```python
from build123d import *

# Parameters (mm, degrees)
SKETCH1_W                 = 254
SKETCH1_H                 = 114.3
BOSS_EXTRUDE1_DEPTH       = 5.08
CHAMFER1_SIZE             = 5.08
BOSS_EXTRUDE3_START       = -127
BOSS_EXTRUDE3_DEPTH       = 38.1
BOSS_EXTRUDE4_DEPTH       = 2.54
SKETCH6_R                 = 3
BOSS_EXTRUDE5_DEPTH       = 6
SKETCH12_R                = 3
SKETCH12_R_2              = 3.5
BOSS_EXTRUDE7_DEPTH       = 6
F_3_0MM_DOWEL_HOLE1_D     = 3
F_3_0MM_DOWEL_HOLE1_DEPTH = 5.08


with BuildPart() as part:
    # Sketch1 → Boss-Extrude1 (new body)
    with BuildSketch(Plane(origin=(0, 0, 0), x_dir=(1, 0, 0), z_dir=(0, 1, 0))):
        with Locations((-127, 57.15)):
            Rectangle(SKETCH1_W, SKETCH1_H)
    extrude(amount=BOSS_EXTRUDE1_DEPTH)

    # Chamfer1
    chamfer1_edges = [part.edges().sort_by_distance(p)[0] for p in [
        (0, 2.54, 0),
        (-254, 2.54, 0),
        (-254, 2.54, -114.3),
        (0, 2.54, -114.3),
    ]]
    chamfer(chamfer1_edges, length=CHAMFER1_SIZE)

    # Sketch3 → Boss-Extrude3 (add, symmetric)
    with BuildSketch(Plane(origin=(0, 0, 0), x_dir=(0, 0, -1), z_dir=(1, 0, 0)).offset(BOSS_EXTRUDE3_START)):
        Polygon((2.667, 5.08), (2.667, 6.35), (2.032, 7.62), (2.667, 8.89), (3.937, 8.89), (3.937, 5.08), align=None)
    boss_extrude3 = extrude(amount=BOSS_EXTRUDE3_DEPTH, both=True)

    # Mirror1: Boss-Extrude3 across plane
    add(boss_extrude3.mirror(Plane.XY.offset(-57.15)))

    # Sketch4 → Boss-Extrude4 (add)
    with BuildSketch(Plane(origin=(0, 5.08, 0), x_dir=(1, 0, 0), z_dir=(0, 1, 0))):
        Polygon((-6.184707571, 111.633), (-247.815292429, 111.633), (-251.333, 108.115292429), (-251.333, 6.184707571), (-247.815292429, 2.667), (-6.184707571, 2.667), (-2.667, 6.184707571), (-2.667, 108.115292429), align=None)
        Polygon((-7.247331044, 109.0676), (-246.752668956, 109.0676), (-248.7676, 107.052668956), (-248.7676, 7.247331044), (-246.752668956, 5.2324), (-7.247331044, 5.2324), (-5.2324, 7.247331044), (-5.2324, 107.052668956), align=None, mode=Mode.SUBTRACT)
    extrude(amount=BOSS_EXTRUDE4_DEPTH)

    # Sketch6 → Boss-Extrude5 (add)
    with BuildSketch(Plane(origin=(0, 5.08, 0), x_dir=(1, 0, 0), z_dir=(0, 1, 0))):
        with Locations((-30.6324, 67.31)):
            Circle(SKETCH6_R)
        with Locations((-30.6324, 19.05)):
            Circle(SKETCH6_R)
        with Locations((-82.7024, 52.07)):
            Circle(SKETCH6_R)
        with Locations((-82.7024, 24.13)):
            Circle(SKETCH6_R)
    extrude(amount=BOSS_EXTRUDE5_DEPTH)

    # Sketch12 → Boss-Extrude7 (add)
    with BuildSketch(Plane(origin=(0, 5.08, 0), x_dir=(1, 0, 0), z_dir=(0, 1, 0))):
        with Locations((-132.2324, 67.4624)):
            Circle(SKETCH12_R)
        with Locations((-132.2324, 11.5824)):
            Circle(SKETCH12_R)
        with Locations((-113.1824, 67.4624)):
            Circle(SKETCH12_R)
        with Locations((-113.1824, 11.5824)):
            Circle(SKETCH12_R)
        with Locations((-81.4324, 96.3676)):
            Circle(SKETCH12_R_2)
        with Locations((-171.4324, 96.3676)):
            Circle(SKETCH12_R_2)
    extrude(amount=BOSS_EXTRUDE7_DEPTH)

    # Ø3.0mm Dowel Hole1
    with Locations(Plane(origin=(0, 11.08, 0), x_dir=(1, 0, 0), z_dir=(0, 1, 0))):
        with Locations((-82.7024, 24.13), (-82.7024, 52.07), (-30.6324, 67.31), (-30.6324, 19.05), (-132.2324, 11.5824), (-113.1824, 11.5824), (-171.4324, 96.3676), (-132.2324, 67.4624), (-113.1824, 67.4624), (-81.4324, 96.3676)):
            Hole(F_3_0MM_DOWEL_HOLE1_D / 2, depth=F_3_0MM_DOWEL_HOLE1_DEPTH)


solid = part.part
```
Part model, mm, in its own coordinate system. A direction names the side the tool comes from. Coordinates: 2 decimals unless noted, no trailing zeros. Write each loop counter-clockwise with the first axis right and the second up, starting at its lowest first coordinate (ties: lowest second). Pieces come first, ordered by that corner, then holes.
Item 1: Slice it at C-C (x = -152.5). Write the cut outline in (y, z).
Item 2: Pin check, flat tips, straight feed: pin 1 (5 mm diameter, centred on x = -149.5, z = -19, fed in from +Y); pin 2 (1 mm diameter, centred on x = -128.5, z = -110.5, fed in from +Y); pin 3 (3 mm diameter, centred on x = -92.5, y = 7, fed in from +Z). Stop position of each tip, or through.
Item 3: Slice it at A-A (z = -104). Write the cut outline in (x, y), and give its area (3 significant figures).
Item 4: Which spindle directions (+Z, -Z, +X, -X, +Y, -Y) get a long thin tool onto all of the face, cutting with end or side? Do faces 5 (the face through (-129, 5.08, -58)), 6 (the face through (-2.5, 2.5, -2.58)). Say none if no direction does.
Item 5: Probe line 1 (X direction, y = 7, z = -37); line 2 (Z direction, x = -212, y = 5.5); line 3 (Z direction, x = -172, y = 7.5). List the from-to ranges inside material, lowest first.
Item 6: Mould opens along Z. For faces 1 (the face through (-251.42, 2.5, -111.8)), 2 (the face through (-115.394, 8.038, -69.49)), 3 (the face through (-33.63, 8.04, -19.18)), 4 (the face through (-169.9, 11.08, -95.6)) say: released by +Z, released by -Z, zero draft, split by the parting line, or undercut.
Item 7: Slice it at B-B (x = -213). Write the cut outline in (y, z), and give its area (3 significant figures).
Results found:
1. outline: (0, -114.3) - (5.08, -114.3) - (5.08, -111.63) - (6.35, -111.63) - (7.62, -112.27) - (8.89, -111.63) - (8.89, -110.36) - (7.62, -110.36) - (7.62, -109.07) - (5.08, -109.07) - (5.08, -5.23) - (7.62, -5.23) - (7.62, -3.94) - (8.89, -3.94) - (8.89, -2.67) - (7.62, -2.03) - (6.35, -2.67) - (5.08, -2.67) - (5.08, 0) - (0, 0) - close
2. pin 1: stops at y = 5.08
2. pin 2: stops at y = 8.89
2. pin 3: stops at z = -2.03
3. outline: (-254, 0) - (0, 0) - (0, 5.08) - (-2.67, 5.08) - (-2.67, 7.62) - (-5.23, 7.62) - (-5.23, 5.08) - (-248.77, 5.08) - (-248.77, 7.62) - (-251.33, 7.62) - (-251.33, 5.08) - (-254, 5.08) - close
3. area: 1,300 mm2
4. face 5: +Y
4. face 6: +Z, +X, +Y, -Y
5. line 1: x = -251.33 to -248.77, -5.23 to -2.67
5. line 2: z = -111.63 to -109.07, -5.23 to -2.67
5. line 3: z = -111.63 to -109.07, -99.82 to -97.76, -94.98 to -92.91, -5.23 to -2.67
6. face 1: released by -Z
6. face 2: undercut
6. face 3: undercut
6. face 4: zero draft
7. outline: (0, -114.3) - (5.08, -114.3) - (5.08, -111.63) - (7.62, -111.63) - (7.62, -109.07) - (5.08, -109.07) - (5.08, -5.23) - (7.62, -5.23) - (7.62, -2.67) - (5.08, -2.67) - (5.08, 0) - (0, 0) - close
7. area: 594 mm2
